Answer from the drawing. Dimensions are ordinates in mm from the lowest x, y and z of the part. A direction names the side the tool comes from. Round coordinates to 2 decimals unless told otherwise and drop trailing zeros. Write each loop counter-clockwise with the first axis right and the second up, starting at its lowest first coordinate (ties: lowest second). Pieces come first, ordered by that corner, then holes. Notation, with made-up numbers: (59, 46) - (117, 46) arc R15 ccw to (117, 71) - close; hole circle Ø10 at (40.5, 63.25). An arc over 180 degrees is marked (long way). Answer as a JSON object with one key per item and string values.
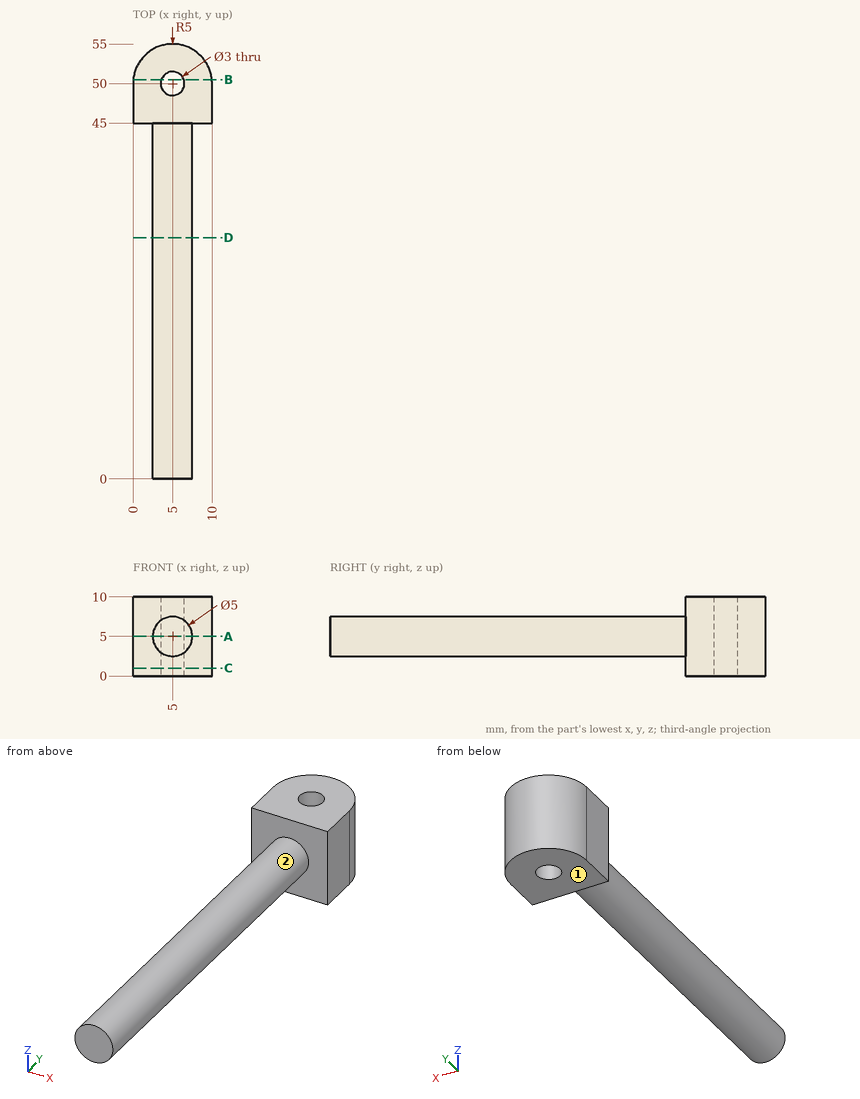
Item 1: A cutting plane is placed at A-A (z = 5). Write down the section's boundary in (x, y), and give its area (3 significant figures).
Results found:
{"outline": "(0, 45) - (2.5, 45) - (2.5, 0) - (7.5, 0) - (7.5, 45) - (10, 45) - (10, 50) arc R5 ccw to (0, 50) - close; hole circle Ø3 at (5, 50)", "area": "307 mm²"}
Item 2: For the marked faces 1 and 2, determine the directions among +Z, -Z, +X, -X, +Y, -Y from which every point of the face is accessible in a straight line to the end or side of a thin tool.
Results found:
{"face 1": "-Z, +X, -X, +Y, -Y", "face 2": "-Y"}
Item 3: A cutting plane is placed at D-D (y = 30.5). Write down the section's boundary in (x, z).
Results found:
{"outline": "circle Ø5 at (5, 5)"}
Item 4: Consider line 1 along Y through (x, z) = (5, 2.75); line 2 along Y through (x, z) = (6.75, 1.75); line 3 along X through (y, z) = (12, 6). Determine where each line is inside the solid, lowest interval first.
Results found:
{"line 1": "0 to 48.5, 51.5 to 55", "line 2": "45 to 54.68", "line 3": "2.71 to 7.29"}
Item 5: A cutting plane is placed at C-C (z = 1). Write down the section's boundary in (x, y).
Results found:
{"outline": "(0, 45) - (10, 45) - (10, 50) arc R5 ccw to (0, 50) - close; hole circle Ø3 at (5, 50)"}
Item 6: A cutting plane is placed at B-B (y = 50.5). Write down the section's boundary in (x, z), and give its area (3 significant figures).
Results found:
{"outline": "(0.03, 0) - (3.59, 0) - (3.59, 10) - (0.03, 10) - close; (6.41, 0) - (9.97, 0) - (9.97, 10) - (6.41, 10) - close", "area": "71.2 mm²"}
Item 7: Each of these flat-tipped pins is pushed along its axis until it touches: P1, Ø4, axis at x = 3, z = 4, coming from the -Y side; P2, Ø5, axis at y = 17, z = 6, coming from the -X side; P3, Ø5, axis at x = 2.5, y = 9.5, coming from the -Z side; P4, Ø1, axis at x = 4, y = 36.5, coming from the +Z side. Where does it stop, or does it pass through?
Results found:
{"P1": "y = 0", "P2": "x = 2.5", "P3": "z = 2.5", "P4": "z = 7.45"}
